Source: CAD feature listing. Evaluate the final solid. Frame: model axes, mm. A direction names the side the tool comes from. Give positions to 0.01 mm unless a question says otherwise; leave off trailing zeros. Write each loop counter-clockwise with the first axis right and the second up, starting at its lowest first coordinate (ties: lowest second). Pieces come first, ordered by that corner, then holes. Notation, with made-up numbers: (-28.5, 9.25) -> (27.5, 9.25) arc R25 ccw to (27.5, 48.25) -> close; hole circle Ø5 at (44.25, 16). An arc over 180 degrees is marked (long way). Answer as a JSON object with one key per item and string values. Group by question number.
Item 1: Section query A-A on z = 12. Return the cut outline in (x, y), plus the area to 3 significant figures.
Item 2: Section query D-D on z = 4.5. Return the cut outline in (x, y), plus the area to 3 significant figures.
Item 3: First-contact query: pin 1 Ø2 at (x, y) = (-6.66, -12.15) entering from +Z; pin 2 Ø6 at (y, z) = (37, 19.5) entering from -X; pin 3 Ø3 at (x, z) = (-1.5, 5.5) entering from -Y. Flat tips, straight axial feed; report the tip coordinate or a pass-through.
Item 4: Ray query, probe 1 along Y at (x, z) = (22.7, 12); probe 2 along X at (y, z) = (-16, 1.2); probe 3 along Z at (x, y) = (16.5, 22). Return the intervals inside material, ascending. Write a range as from..to.
Item 5: Pull-direction query (X, two-part tool) for faces 1 (the face through (-7.218, -19.341, 1.521)), 2 (the face through (0, -25, 1)), 3 (the face through (-3.104, -9.237, 1.521)), 4 (the face through (7, -24, 2)); classes: pulls with the +X half, pulls with the -X half, needs draft (parallel to the pull), parting line crosses it, or undercut.
Item 6: Section query B-B on y = -16. Return the cut outline in (x, z), plus the area to 3 significant figures.
Item 7: Section query C-C on y = 7. Return the cut outline in (x, z).
Item 8: Access query for faces 5 (the face through (8, 23, 2)), 6 (the face through (9, 0, 1)), 7 (the face through (12.9, 5, 8.6)). Directions: +Z, -Z, +X, -X, +Y, -Y. A direction counts if a zero-diameter tool reaches every point of the face in a straight line with its end or side. Return the directions, or none.
Autodesk Inventor part; units mm, degrees
ref_plane "YZ Plane" through (0, 0, 0) normal (1, 0, 0) x (0, 1, 0)
ref_plane "XZ Plane" through (0, 0, 0) normal (0, 1, 0) x (-1, 0, 0)
ref_plane "XY Plane" through (0, 0, 0) normal (0, 0, 1) x (1, 0, 0)
sketch "Sketch1" plane through (0, 0, 0) normal (0, 0, 1) x (1, 0, 0)
  line L0 (-9, 25) -> (9, 25)
  line L1 (9, 25) -> (9, -25)
  line L2 (9, -25) -> (-9, -25)
  line L3 (-9, -25) -> (-9, 25)
  point P0 (0, 0)
  point P1 (0, 25)
  point P2 (-9, 0)
  dimension "d0" = 18
  dimension "d1" = 50
extrude "Extrusion1" add sketch "Sketch1" along normal blind 3
fillet "Fillet1" radius 5 2 edges at (-9, -25, 1.5) (9, -25, 1.5)
fillet "Fillet2" radius 5 2 edges at (-9, 25, 1.5) (9, 25, 1.5)
sketch "Sketch2" plane through (0, 0, 3) normal (0, 0, 1) x (1, 0, 0)
  circle A0 centre (0, -16) radius 9
  circle A1 centre (0, 16) radius 9
  line L0 (-4, -25) -> (4, -25)
  circle A2 centre (0, -8.304) radius 0.75
  line L1 (4, 25) -> (-4, 25)
  point P0 (0, 0)
  dimension "d6" = 18
  dimension "d8" = 1.5
  dimension "d10" = 18
extrude "Extrusion2" cut sketch "Sketch2" against normal up to surface (3 mm away) contours A2
pattern_circular "Circular Pattern1" count 12 over 360 about axis through (0, -16, 3) along (0, 0, 1) of "Extrusion2"
sketch "Sketch4" plane through (0, 0, 3) normal (0, 0, 1) x (1, 0, 0)
  line L0 (-9, 5) -> (27, 5)
  line L1 (27, 5) -> (27, 50)
  line L2 (27, 50) -> (-9, 50)
  line L3 (-9, 50) -> (-9, 5)
  line L4 (-9, 20) -> (-9, -20)
  line L5 (4, 25) -> (-4, 25)
  point P0 (0, 0)
  dimension "d25" = 36
  dimension "d26" = 45
  dimension "d27" = 20
extrude "Extrusion5" add sketch "Sketch4" along normal blind 6
sketch "Sketch5" plane through (0, 0, 3) normal (0, 0, 1) x (1, 0, 0)
  line L0 (27, 50) -> (-9, 50)
  line L1 (27, 5) -> (21, 5)
  line L2 (21, 5) -> (21, 50)
  line L3 (21, 50) -> (27, 50)
  line L4 (27, 50) -> (27, 5)
  point P0 (0, 0)
  dimension "d30" = 6
extrude "Extrusion6" add sketch "Sketch5" along normal blind 28
sketch "Sketch6" plane through (21, 5, 3) normal (-1, 0, 0) x (0, 0, 1)
  circle A0 centre (25, 4) radius 1
  circle A1 centre (9, 4) radius 1
  circle A2 centre (25, 41) radius 1
  circle A3 centre (9, 41) radius 1
  line L0 (6, 0) -> (28, 0)
  line L1 (25, 4) -> (25, 41) construction
  line L2 (28, 45) -> (28, 0)
  point P0 (-3, -5)
  point P1 (0, 0)
  point P2 (28, 22.5)
  point P3 (25, 22.5)
  dimension "d33" = 2
  dimension "d34" = 2
  dimension "d35" = 2
  dimension "d36" = 2
  dimension "d37" = 37
  dimension "d38" = 16
  dimension "d40" = 16
  dimension "d43" = 3
extrude "Extrusion7" cut sketch "Sketch6" against normal up to surface (6 mm away)
properties part number "first_perc_link"
Worked answers:
{
 "1": {"outline": "(21, 5) -> (27, 5) -> (27, 8) -> (21, 8) -> close; (21, 10) -> (27, 10) -> (27, 45) -> (21, 45) -> close; (21, 47) -> (27, 47) -> (27, 50) -> (21, 50) -> close", "area": "246 mm^2"},
 "2": {"outline": "(-9, 5) -> (27, 5) -> (27, 50) -> (-9, 50) -> close", "area": "1,620 mm^2"},
 "3": {"pin 1": "z = 3", "pin 2": "x = 21", "pin 3": "y = 5"},
 "4": {"probe 1": "5..8, 10..45, 47..50", "probe 2": "-9..-8.45, -6.95..6.95, 8.45..9", "probe 3": "3..9"},
 "5": {"face 1": "undercut", "face 2": "needs draft", "face 3": "undercut", "face 4": "pulls with the +X half"},
 "6": {"outline": "(-9, 0) -> (-8.45, 0) -> (-8.45, 3) -> (-9, 3) -> close; (-6.95, 0) -> (6.95, 0) -> (6.95, 3) -> (-6.95, 3) -> close; (8.45, 0) -> (9, 0) -> (9, 3) -> (8.45, 3) -> close", "area": "45.0 mm^2"},
 "7": {"outline": "(-9, 0) -> (9, 0) -> (9, 3) -> (27, 3) -> (27, 31) -> (21, 31) -> (21, 9) -> (-9, 9) -> close"},
 "8": {"face 5": "-Z, +X, +Y", "face 6": "-Z, +X, +Y, -Y", "face 7": "+Z, +X, -X, -Y"}
}
